Part model, mm, in its own coordinate system. A direction names the side the tool comes from. Coordinates: 2 decimals unless noted, no trailing zeros. Order: outer loops, then holes, each group sorted by start corner. A loop starts at its lowest first (then second) coordinate and runs counter-clockwise, first axis right, second up.
from build123d import *

# Parameters (mm, degrees)
ESBO_O1_W                   = 110
ESBO_O1_H                   = 250
RESSALTO_EXTRUS_O1_DEPTH    = 1.5
FURO_COM_FOLGA_DE_M62_D     = 6.6
FURO_COM_FOLGA_DE_M62_DEPTH = 10
FURO_COM_FOLGA_DE_M62_TIP   = 1.982840043
DOBRA_START                 = -55
DOBRA_ESBO_ADA1_DEPTH       = 110
DOBRA_ESBO_ADA1_2_DEPTH     = 110
DOBRA_ESBO_ADA2_DEPTH       = 110
DOBRA_ESBO_ADA2_2_DEPTH     = 110
ESBO_O12_W                  = 30
ESBO_O12_H                  = 63
CORTE_EXTRUS_O1_DEPTH       = 10


# Read off the part's stored shape, not the designer's step: Dobra esboçada1, Dobra esboçada2
with BuildPart() as part:
    # Esboço1 → Ressalto-extrusão1 (new body)
    with BuildSketch(Plane.XY):
        Rectangle(ESBO_O1_W, ESBO_O1_H)
    extrude(amount=RESSALTO_EXTRUS_O1_DEPTH)

    # Furo com folga de M62
    with Locations(Plane.XY.offset(1.5)):
        with Locations((0, 51), (-44.6, 0), (44.6, 0), (11.3, -37.5)):
            Hole(FURO_COM_FOLGA_DE_M62_D / 2, depth=FURO_COM_FOLGA_DE_M62_DEPTH)
            with Locations((0, 0, -(FURO_COM_FOLGA_DE_M62_DEPTH + FURO_COM_FOLGA_DE_M62_TIP / 2))):  # 118° drill point
                Cone(0, FURO_COM_FOLGA_DE_M62_D / 2, FURO_COM_FOLGA_DE_M62_TIP, mode=Mode.SUBTRACT)

    # Dobra esboçada1 outline → Dobra esboçada1 (cut)
    with BuildSketch(Plane.YZ.offset(DOBRA_START)):
        with BuildLine():
            ThreePointArc((-77.840155051, 0), (-79.460340225, 0.397581589), (-80.712436374, 1.5))
            Line((-80.712436374, 1.5), (-125, 1.5))
            Line((-125, 1.5), (-125, 0))
            Line((-125, 0), (-77.840155051, 0))
        make_face()
    extrude(amount=DOBRA_ESBO_ADA1_DEPTH, mode=Mode.SUBTRACT)

    # Dobra esbo_ada1 2 outline → Dobra esbo_ada1 2 (add)
    with BuildSketch(Plane.YZ.offset(DOBRA_START)):
        with BuildLine():
            ThreePointArc((-77.840155051, 1.5), (-79.254368613, 2.085786438), (-79.840155051, 3.5))
            Line((-79.840155051, 3.5), (-79.840155051, 46.340155051))
            Line((-79.840155051, 46.340155051), (-81.340155051, 46.340155051))
            Line((-81.340155051, 46.340155051), (-81.340155051, 3.5))
            ThreePointArc((-81.340155051, 3.5), (-81.179540071, 2.451902827), (-80.712436374, 1.5))
            Line((-80.712436374, 1.5), (-77.840155051, 1.5))
        make_face()
    extrude(amount=DOBRA_ESBO_ADA1_2_DEPTH)

    # Dobra esboçada2 outline → Dobra esboçada2 (cut)
    with BuildSketch(Plane.YZ.offset(DOBRA_START)):
        with BuildLine():
            Line((125, 1.5), (80.712436374, 1.5))
            ThreePointArc((80.712436374, 1.5), (79.460340225, 0.397581589), (77.840155051, 0))
            Line((77.840155051, 0), (125, 0))
            Line((125, 0), (125, 1.5))
        make_face()
    extrude(amount=DOBRA_ESBO_ADA2_DEPTH, mode=Mode.SUBTRACT)

    # Dobra esbo_ada2 2 outline → Dobra esbo_ada2 2 (add)
    with BuildSketch(Plane.YZ.offset(DOBRA_START)):
        with BuildLine():
            Line((81.340155051, 3.5), (81.340155051, 46.340155051))
            Line((81.340155051, 46.340155051), (79.840155051, 46.340155051))
            Line((79.840155051, 46.340155051), (79.840155051, 3.5))
            ThreePointArc((79.840155051, 3.5), (79.254368613, 2.085786438), (77.840155051, 1.5))
            Line((77.840155051, 1.5), (80.712436374, 1.5))
            ThreePointArc((80.712436374, 1.5), (81.179540071, 2.451902827), (81.340155051, 3.5))
        make_face()
    extrude(amount=DOBRA_ESBO_ADA2_2_DEPTH)

    # Esboço12 → Corte-extrusão1 (cut)
    with BuildSketch(Plane(origin=(0, 0, 0), x_dir=(-1, 0, 0), z_dir=(0, 0, -1))):
        with Locations((40, 36.5)):
            Rectangle(ESBO_O12_W, ESBO_O12_H)
    extrude(amount=-CORTE_EXTRUS_O1_DEPTH, mode=Mode.SUBTRACT)


solid = part.part
Q1. Cut at C-C on y = 0. Write the cut outline in (x, z).
Results list:
outline: (-55, 0) - (-47.9, 0) - (-47.9, 1.5) - (-55, 1.5) - close; (-41.3, 0) - (41.3, 0) - (41.3, 1.5) - (-41.3, 1.5) - close; (47.9, 0) - (55, 0) - (55, 1.5) - (47.9, 1.5) - close
Q2. Mould opens along Y. For faces 1 (the face through (-55, -58, 1)), 2 (the face through (-1, 1, 1.5)), 3 (the face through (-1, -81.34, 25)) say: pulls with the +Y half, pulls with the -Y half, needs draft (parallel to the pull), parting line crosses it, or undercut.
Results list:
face 1: needs draft
face 2: undercut
face 3: pulls with the -Y half
Q3. Pin check, flat tips, straight feed: pin 1 Ø1.6 at (x, z) = (-35, 1) entering from +Y; pin 2 Ø6 at (x, y) = (43, -17.5) entering from +Z; pin 3 Ø1.6 at (y, z) = (38, 0.5) entering from -X. Stop position of each tip, or through.
Results list:
pin 1: stops at y = 80.9
pin 2: stops at z = 1.5
pin 3: stops at x = -25
Q4. Cut at D-D on z = 10. Write the cut outline in (x, y), and give its area (3 significant figures).
Results list:
outline: (-55, -81.34) - (55, -81.34) - (55, -79.84) - (-55, -79.84) - close; (-55, 79.84) - (55, 79.84) - (55, 81.34) - (-55, 81.34) - close
area: 330 mm2
Q5. Cut at A-A on x = -36. Write the cut outline in (y, z), and give its area (4 significant figures).
Results list:
outline: (-81.34, 3.5) arc R3.5 ccw to (-77.84, 0) - (5, 0) - (5, 1.5) - (-77.84, 1.5) arc R2 cw to (-79.84, 3.5) - (-79.84, 46.34) - (-81.34, 46.34) - close; (68, 0) - (77.84, 0) arc R3.5 ccw to (81.34, 3.5) - (81.34, 46.34) - (79.84, 46.34) - (79.84, 3.5) arc R2 cw to (77.84, 1.5) - (68, 1.5) - close
area: 280.5 mm2
Q6. Which spindle directions (+Z, -Z, +X, -X, +Y, -Y) get a long thin tool onto all of the face, cutting with end or side? Do faces 4 (the face through (9.526, -34.717, 0.739)), 5 (the face through (-1, -79.84, 25)). Say none if no direction does.
Results list:
face 4: +Z, -Z
face 5: +Z, +X, -X
Q7. Cut at B-B on y = -37.5. Write the cut outline in (x, z), and give its area (3 significant figures).
Results list:
outline: (-55, 0) - (8, 0) - (8, 1.5) - (-55, 1.5) - close; (14.6, 0) - (55, 0) - (55, 1.5) - (14.6, 1.5) - close
area: 155 mm2
Q8. Wall check: line 1 along Y through (x, z) = (1.5, 35); line 2 along Z through (x, y) = (49, 19.5); line 3 along Y through (x, z) = (0, 0.55). Give the ranges that are in metal, low to high.
Results list:
line 1: y = -81.34 to -79.84, 79.84 to 81.34
line 2: z = 0 to 1.5
line 3: y = -79.72 to 47.7, 54.3 to 79.72
